from build123d import *

# Parameters (mm, degrees)
F0_W     = 159.6704572439
F0_H     = 91.4154052735
F1_DEPTH = 81.026
F3_DEPTH = 159.6714572439
F5_DEPTH = 60.6369841733


with BuildPart() as f1:
    # F0 (on Front) → F1 (new body)
    with BuildSketch(Plane.XZ):
        with Locations((-5.7597234845, -5.4780766368)):
            Rectangle(F0_W, F0_H)
    extrude(amount=F1_DEPTH)

    # F2 (on face) → F3 (cut, through all)
    with BuildSketch(Plane.YZ.offset(74.0755051374)):
        Polygon((-81.026, -51.1857792735), (0, 40.229626), (-81.026, 40.229626), align=None)
    extrude(amount=-F3_DEPTH, mode=Mode.SUBTRACT)

    # F4 (on face) → F5 (cut, through all)
    with BuildSketch(Plane(origin=(0, -19.9693104316, 17.699788588), x_dir=(1, 0, 0), z_dir=(0, -0.7483521854, 0.6633015955))):
        Polygon((74.0755051374, 30.1059285345), (-85.5949521065, 30.1059285345), (74.0755051374, -92.049664859), align=None)
    extrude(amount=-F5_DEPTH, mode=Mode.SUBTRACT)


solid = f1.part
Model file for the job. Use its own axes, mm. Give positions to 0.01 mm unless a question says otherwise; leave off trailing zeros. Order: outer loops, then holes, each group sorted by start corner. A loop starts at its lowest first (then second) coordinate and runs counter-clockwise, first axis right, second up. Notation, with made-up numbers: (87, 3) - (123, 3) arc R12 ccw to (123, 21) - close; hole circle Ø4 at (6, 26). An arc over 180 degrees is marked (long way). One line per item, written item: value.
Item 1: Slice it at C-C (z = -19.5). List the corners of the cut face in (x, y).
Response values:
outline: (-85.59, -52.94) - (18.73, -52.94) - (-27.17, 0) - (-85.59, 0) - close
Item 2: Pin check, flat tips, straight feed: pin 1 Ø12 at (x, y) = (17, -21.5) entering from +Z; pin 2 Ø3 at (y, z) = (-10, -26.5) entering from +X; pin 3 Ø6 at (x, y) = (-20.5, -36.5) entering from +Z. Stop position of each tip, or through.
Response values:
pin 1: z = -37.48
pin 2: x = -9.69
pin 3: z = 2.43
Item 3: Wall check: line 1 (X direction, y = -29, z = -27); line 2 (X direction, y = -30.5, z = -2); line 3 (Z direction, x = -53, y = -27). Give the ranges that are in metal, low to high.
Response values:
line 1: -85.59 to 5.31
line 2: -85.59 to -17.84
line 3: -51.19 to 9.77
Item 4: Slice it at B-B (x = 35). List the corners of the cut face in (y, z), then the cut area to 3 significant figures.
Response values:
outline: (-81.03, -51.19) - (-35.96, -51.19) - (-61.2, -28.81) - close
area: 504 mm2
Item 5: Slice it at A-A (y = -64). List the corners of the cut face in (x, z).
Response values:
outline: (-85.59, -51.19) - (59.31, -51.19) - (40.52, -31.98) - (-85.59, -31.98) - close
Item 6: Slice it at D-D (x = 53.5). List the corners of the cut face in (y, z), then the cut area to 3 significant figures.
Response values:
outline: (-81.03, -51.19) - (-57.29, -51.19) - (-70.58, -39.41) - close
area: 140 mm2
